Geometry check sheet. Reference: the model listing, model coordinates, mm. A direction names the side the tool comes from. Round coordinates to 2 decimals unless told otherwise and drop trailing zeros. Loops run counter-clockwise (first coordinate to the right, second up) from the corner with the lowest first, then second, coordinate; pieces in that order, holes last. Notation, with made-up numbers: (62, 29.5) - (72, 29.5) arc R9 ccw to (72, 41.5) - close; hole circle Ø3 at (-29.75, -7). An arc over 180 degrees is marked (long way). Answer in a Markdown table with one row per item. Add a question column.
Autodesk Inventor part; units mm, degrees
ref_plane "YZ Plane" through (0, 0, 0) normal (1, 0, 0) x (0, 1, 0)
ref_plane "XZ Plane" through (0, 0, 0) normal (0, 1, 0) x (-1, 0, 0)
ref_plane "XY Plane" through (0, 0, 0) normal (0, 0, 1) x (1, 0, 0)
sketch "スケッチ1" plane through (0, 0, 0) normal (0, 0, 1) x (1, 0, 0)
  circle A0 centre (0, 0) radius 1.25
  circle A1 centre (0, 0) radius 5
  line L0 (-10, -6) -> (10, -6)
  line L1 (10, -6) -> (10, -9)
  line L2 (10, -9) -> (-10, -9)
  line L3 (-10, -9) -> (-10, -6)
  line L4 (-5, 0) -> (-5, -6)
  line L5 (5, 0) -> (5, -6)
  circle A2 centre (-5.7106, -5.2894) radius 1.005
  circle A3 centre (5.7106, -5.2894) radius 1.005
  line L6 (-5.7106, -5.2894) -> (-5, -6)
  line L7 (5.7106, -5.2894) -> (5, -6)
  point P0 (6.4213, -6)
  point P1 (5, -4.5787)
  point P2 (-5, -4.5787)
  point P3 (-6.4213, -6)
  dimension "d7" = 2.01
  dimension "d8" = 2.01
  dimension "d0" = 2.5
  dimension "d1" = 10
  dimension "d2" = 3
  dimension "d3" = 20
  dimension "d4" = 6
  dimension "d5" = 5
  dimension "d6" = 6
  dimension "d9" = 45
  dimension "d10" = 45
extrude "押し出し1" add sketch "スケッチ1" along normal blind 3 contours A1 | L5 A3 L0 A2 L4 A1 | A3 L0 L1 L2 L3 A2
thread "ねじ1"
sketch "スケッチ2" plane through (0, 0, 3) normal (0, 0, 1) x (1, 0, 0)
  line L0 (-10, -6) -> (-10, -9)
  line L1 (-10, -9) -> (10, -9)
  line L2 (10, -9) -> (10, -6)
  line L3 (10, -6) -> (6.4213, -6)
  arc A0 (5, -4.5787) -> (6.4213, -6) centre (5.7106, -5.2894) ccw
  line L4 (5, -4.5787) -> (5, 0)
  arc A1 (5, 0) -> (-5, 0) centre (0, 0) ccw
  line L5 (-5, 0) -> (-5, -4.5787)
  arc A2 (-6.4213, -6) -> (-5, -4.5787) centre (-5.7106, -5.2894) ccw
  line L6 (-6.4213, -6) -> (-10, -6)
  circle A3 centre (0, 0) radius 1.25
properties part number "T字金具M3" material "アルミニウム 7075"
Q1. Cross-section at D-D, the plane x = 6.75. Enter the section's corners in (y, z), plus the area to 3 significant figures.
Q2. Cross-section at B-B, the plane y = -1. Enter the section's corners in (x, z), plus the area to 3 significant figures.
Q3. Cross-section at C-C, the plane x = 0. Enter the section's corners in (y, z), plus the area to 3 significant figures.
Q4. Scan lines: line 1 (Y direction, x = 0, z = 1.85); line 2 (X direction, y = -1.5, z = 0.35); line 3 (Y direction, x = 7.5, z = 1.85). Record each from-to range of solid material in increasing order. Write a range as from..to.
Q5. Set-up check for faces 4 (the flat face through (5, -2, 1)), 5 (the flat face through (-5, -2, 1)), 6 (the cylindrical face through (5, -6, 1)): record each of +Z, -Z, +X, -X, +Y, -Y from which the full face is reachable in a straight line by a thin tool's end or side.
Q6. Depth check by flat-ended pin: P1, Ø0.9, axis at y = -3.5, z = 1, coming from the -X side; P2, Ø0.9, axis at x = -8, z = 2, coming from the +Y side. Enter the tip coordinate at first touch or a pass-through.
Q7. Cross-section at A-A, the plane z = 1.8. Enter the section's corners in (x, y) (3 decimals), plus the area to 3 significant figures.
Q8. Release check for a two-part mould opening along X. For faces 1 (the cylindrical face through (-5, -6, 1)), 2 (the cylindrical face through (0, 5, 1)), 3 (the flat face through (0, -3, 0)) record: +X half, -X half, draft (parallel to the pull), parting line (faces both ways), or undercut.
Check sheet entries:
| question | item | result |
|---|---|---|
| 1 | outline | (-9, 0) - (-6, 0) - (-6, 3) - (-9, 3) - close |
| 1 | area | 9.00 mm² |
| 2 | outline | (-5, 0) - (-0.75, 0) - (-0.75, 3) - (-5, 3) - close; (0.75, 0) - (5, 0) - (5, 3) - (0.75, 3) - close |
| 2 | area | 25.5 mm² |
| 3 | outline | (-9, 0) - (-1.25, 0) - (-1.25, 3) - (-9, 3) - close; (1.25, 0) - (5, 0) - (5, 3) - (1.25, 3) - close |
| 3 | area | 34.5 mm² |
| 4 | line 1 | -9..-1.25, 1.25..5 |
| 4 | line 2 | -5..5 |
| 4 | line 3 | -9..-6 |
| 5 | face 4 | +Z, -Z, +X, +Y |
| 5 | face 5 | +Z, -Z, -X, +Y |
| 5 | face 6 | +Z, -Z |
| 6 | P1 | x = -5 |
| 6 | P2 | y = -6 |
| 7 | outline | (-10, -9) - (10, -9) - (10, -6) - (6.421, -6) arc R1.005 cw to (5, -4.579) - (5, 0) arc R5 ccw to (-5, 0) - (-5, -4.579) arc R1.005 cw to (-6.421, -6) - (-10, -6) - close; hole circle Ø2.5 at (0, 0) |
| 7 | area | 153 mm² |
| 8 | face 1 | undercut |
| 8 | face 2 | parting line |
| 8 | face 3 | draft |
